Check sheet for the modelled part. Datum: model origin and axes. Units: mm. Round coordinates to 2 decimals unless told otherwise and drop trailing zeros. Write each loop counter-clockwise with the first axis right and the second up, starting at its lowest first coordinate (ties: lowest second). Pieces come first, ordered by that corner, then holes.
Item 1: Cross-section at B-B on z = 3. Enter the section's corners in (x, y).
Item 2: Go/stop test with flat-tipped pins: pin 1 Ø12 at (x, z) = (14.5, -18.5) entering from -Y; pin 2 Ø2.5 at (x, z) = (15.5, 15.5) entering from +Y; pin 3 Ø5 at (x, z) = (40, -23.1) entering from -Y; pin 4 Ø2 at (y, z) = (4.5, -12) entering from -X. Record where each tip stops, or that it passes through.
Item 3: Cross-section at C-C on z = -15.5. Enter the section's corners in (x, y), plus the area to 3 significant figures.
Item 4: Material ranges on line 1 (Z direction, x = 0, y = 1); line 2 (Z direction, x = 15.5, y = 1.1); line 3 (Z direction, x = 12, y = 3.55), recorded low to high.
Item 5: Cross-section at D-D on x = 1. Enter the section's corners in (y, z).
Item 6: Cross-section at A-A on y = 4.1. Count the separate pieces of the cut face and the enclosed holes in it, plus the area to 3 significant figures.
from build123d import *

# Parameters (mm, degrees)
SKETCH2_W                                        = 130
SKETCH2_H                                        = 130
BOSS_EXTRUDE1_DEPTH                              = 5
SKETCH3_R                                        = 13.5
CUT_EXTRUDE1_DEPTH                               = 5
SKETCH8_W                                        = 130
SKETCH8_H                                        = 130
CUT_EXTRUDE6_DEPTH                               = 6
M4_CLEARANCE_HOLE1_D                             = 4.8
M4_CLEARANCE_HOLE1_DEPTH                         = 5
CBORE_FOR_M3_HEX_HEAD_MACHINE_SCREW1_D           = 3.4
CBORE_FOR_M3_HEX_HEAD_MACHINE_SCREW1_DEPTH       = 5
CBORE_FOR_M3_HEX_HEAD_MACHINE_SCREW1_CBORE_D     = 8.4
CBORE_FOR_M3_HEX_HEAD_MACHINE_SCREW1_CBORE_DEPTH = 3.3
CBORE_FOR_M4_SBHCS1_D                            = 4.5
CBORE_FOR_M4_SBHCS1_DEPTH                        = 5
CBORE_FOR_M4_SBHCS1_CBORE_D                      = 8.6
CBORE_FOR_M4_SBHCS1_CBORE_DEPTH                  = 2.2


with BuildPart() as part:
    # Sketch2 → Boss-Extrude1 (new body)
    with BuildSketch(Plane(origin=(0, 0, 0), x_dir=(1, 0, 0), z_dir=(0, 1, 0))):
        Rectangle(SKETCH2_W, SKETCH2_H)
    extrude(amount=BOSS_EXTRUDE1_DEPTH)

    # Sketch3 → Cut-Extrude1 (cut)
    with BuildSketch(Plane(origin=(0, 5, 0), x_dir=(1, 0, 0), z_dir=(0, 1, 0))):
        Circle(SKETCH3_R)
    extrude(amount=-CUT_EXTRUDE1_DEPTH, mode=Mode.SUBTRACT)

    # Sketch8 → Cut-Extrude6 (cut, through all)
    with BuildSketch(Plane(origin=(0, 5, 0), x_dir=(1, 0, 0), z_dir=(0, 1, 0))):
        Rectangle(SKETCH8_W, SKETCH8_H)
        with BuildLine():
            Line((-42.00982343, 32.5), (42.00982343, 32.5))
            ThreePointArc((42.00982343, 32.5), (50.201409492, 28.235670649), (51.406671379, 19.079583559))
            Line((51.406671379, 19.079583559), (25.74494306, -51.420416441))
            ThreePointArc((25.74494306, -51.420416441), (22.083765761, -56.191586062), (16.348095112, -58))
            Line((16.348095112, -58), (-16.348095112, -58))
            ThreePointArc((-16.348095112, -58), (-22.083765761, -56.191586062), (-25.74494306, -51.420416441))
            Line((-25.74494306, -51.420416441), (-51.406671379, 19.079583559))
            ThreePointArc((-51.406671379, 19.079583559), (-50.201409492, 28.235670649), (-42.00982343, 32.5))
        make_face(mode=Mode.SUBTRACT)
    extrude(amount=-CUT_EXTRUDE6_DEPTH, mode=Mode.SUBTRACT)

    # M4 Clearance Hole1
    with Locations(Plane(origin=(0, 5, 0), x_dir=(1, 0, 0), z_dir=(0, 1, 0))):
        with Locations((-27, 24), (27, 24), (27, -24), (-27, -24)):
            Hole(M4_CLEARANCE_HOLE1_D / 2, depth=M4_CLEARANCE_HOLE1_DEPTH)

    # CBORE for M3 Hex Head Machine Screw1
    with Locations(Plane(origin=(0, 5, 0), x_dir=(1, 0, 0), z_dir=(0, 1, 0))):
        with Locations((-15.5, 15.5), (15.5, 15.5), (15.5, -15.5), (-15.5, -15.5)):
            CounterBoreHole(CBORE_FOR_M3_HEX_HEAD_MACHINE_SCREW1_D / 2, CBORE_FOR_M3_HEX_HEAD_MACHINE_SCREW1_CBORE_D / 2, CBORE_FOR_M3_HEX_HEAD_MACHINE_SCREW1_CBORE_DEPTH, depth=CBORE_FOR_M3_HEX_HEAD_MACHINE_SCREW1_DEPTH)

    # CBORE for M4 SBHCS1
    with Locations(Plane(origin=(0, 0, 0), x_dir=(-1, 0, 0), z_dir=(0, -1, 0))):
        with Locations((0, -46.19), (40, 23.1), (-40, 23.1)):
            CounterBoreHole(CBORE_FOR_M4_SBHCS1_D / 2, CBORE_FOR_M4_SBHCS1_CBORE_D / 2, CBORE_FOR_M4_SBHCS1_CBORE_DEPTH, depth=CBORE_FOR_M4_SBHCS1_DEPTH)


solid = part.part
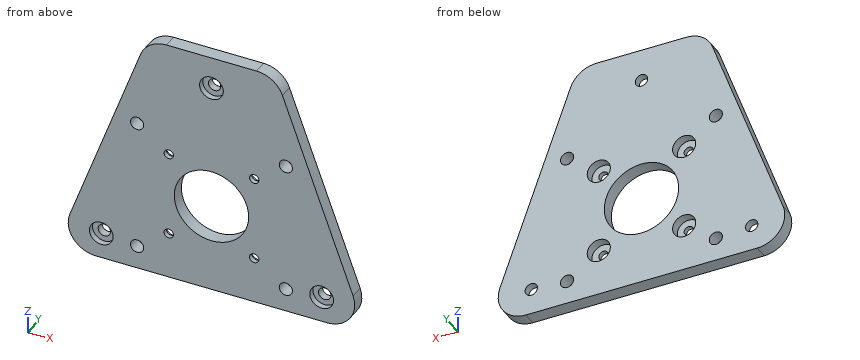
Response values:
1. outline: (-43.37, 0) - (-13.16, 0) - (-13.16, 5) - (-43.37, 5) - close; (13.16, 0) - (43.37, 0) - (43.37, 5) - (13.16, 5) - close
2. pin 1: stops at y = 0
2. pin 2: passes through
2. pin 3: stops at y = 2.2
2. pin 4: stops at x = -49.19
3. outline: (-50.1, 0) - (-17.2, 0) - (-17.2, 1.7) - (-19.7, 1.7) - (-19.7, 5) - (-50.1, 5) - close; (-13.8, 0) - (13.8, 0) - (13.8, 1.7) - (11.3, 1.7) - (11.3, 5) - (-11.3, 5) - (-11.3, 1.7) - (-13.8, 1.7) - close; (17.2, 0) - (50.1, 0) - (50.1, 5) - (19.7, 5) - (19.7, 1.7) - (17.2, 1.7) - close
3. area: 434 mm2
4. line 1: z = -32.5 to -13.5, 13.5 to 41.89, 50.49 to 58
4. line 2: z = -32.5 to -17.2, -13.8 to 13.8, 17.2 to 58
4. line 3: z = -32.5 to -17.82, -13.18 to -6.18, 6.18 to 13.18, 17.82 to 58
5. outline: (0, -32.5) - (5, -32.5) - (5, -13.46) - (0, -13.46) - close; (0, 13.46) - (5, 13.46) - (5, 44.17) - (2.2, 44.17) - (2.2, 42.01) - (0, 42.01) - close; (0, 50.37) - (2.2, 50.37) - (2.2, 48.21) - (5, 48.21) - (5, 58) - (0, 58) - close
6. separate pieces: 1
6. enclosed holes: 12
6. area: 6,180 mm2
